```python
from build123d import *

# Parameters (mm, degrees)
SKETCH1_W           = 390
SKETCH1_H           = 756.8
BOSS_EXTRUDE1_DEPTH = 20
SKETCH2_R           = 6.05
BOSS_EXTRUDE2_DEPTH = 10
SKETCH3_R           = 6.631048811
BOSS_EXTRUDE3_DEPTH = 10
CHAMFER1_SIZE       = 10
BOSS_EXTRUDE5_DEPTH = 50
SKETCH5_W           = 30
SKETCH5_H           = 160
CUT_EXTRUDE1_DEPTH  = 50
CHAMFER2_SIZE       = 10


with BuildPart() as part:
    # Sketch1 → Boss-Extrude1 (new body)
    with BuildSketch(Plane.XY):
        with Locations((154.409313495, -346.327898551)):
            Rectangle(SKETCH1_W, SKETCH1_H)
    extrude(amount=BOSS_EXTRUDE1_DEPTH)

    # Sketch2 → Boss-Extrude2 (add)
    with BuildSketch(Plane(origin=(0, 32.072101449, 0), x_dir=(1, 0, 0), z_dir=(0, 1, 0))):
        with Locations(Location((-28.78378628, -10.435138004, 0), (0, 0, 90))):
            Circle(SKETCH2_R)
    extrude(amount=BOSS_EXTRUDE2_DEPTH)

    # Sketch3 → Boss-Extrude3 (add)
    with BuildSketch(Plane.XZ.offset(724.727898551)):
        with Locations(Location((-28.78378628, 10.435138004, 0), (0, 0, 90))):
            Circle(SKETCH3_R)
    extrude(amount=BOSS_EXTRUDE3_DEPTH)

    # Chamfer1
    # the kernel refuses this chamfer: 10 mm, written as the material it takes off along each edge
    with BuildSketch(Plane(origin=(-40.590686505, -750.44472843, 20), x_dir=(-0.027495876610586317, 0, -0.9996219169112968), z_dir=(0, 1, 0)), Plane(origin=(349.409313495, 57.788931329, 0), x_dir=(-0.9996219169112968, 0, -0.027495876610586334), z_dir=(0, -1, 0))) as chamfer1_piece_1:
        Polygon((CHAMFER1_SIZE * 0.999621916911, -CHAMFER1_SIZE * 0.0274958766106), (-CHAMFER1_SIZE * 0.0274958766106, -CHAMFER1_SIZE * 0.999621916911), (0, 0), align=None)
    extrude(amount=808.233659759, mode=Mode.SUBTRACT)
    with BuildSketch(Plane(origin=(375.126143374, -724.727898551, 20), x_dir=(0, 0.9996219169112968, 0.02749587661058643), z_dir=(-1, 0, 0))) as chamfer1_piece_2_section:
        Polygon((CHAMFER1_SIZE * 0.999621916911, CHAMFER1_SIZE * 0.0274958766106), (-CHAMFER1_SIZE * 0.0274958766106, CHAMFER1_SIZE * 0.999621916911), (0, 0), align=None)
    chamfer1_piece_2 = extrude(amount=441.433659759, mode=Mode.PRIVATE)
    chamfer1_piece_2 = chamfer1_piece_2 - Plane(origin=(-28.78378628, -721.415314621, 10.435138004), x_dir=(0, 0, 1), z_dir=(0, 1, 0)) * Cylinder(6.631048811, 923, mode=Mode.PRIVATE)
    add(chamfer1_piece_2, mode=Mode.SUBTRACT)
    with BuildSketch(Plane(origin=(349.409313495, 57.788931329, 20), x_dir=(-0.9996219169112968, 0, 0.027495876610586282), z_dir=(0, -1, 0)), Plane(origin=(-40.590686505, -750.44472843, 0), x_dir=(-0.027495876610586317, 0, 0.9996219169112968), z_dir=(0, 1, 0))) as chamfer1_piece_3:
        Polygon((CHAMFER1_SIZE * 0.999621916911, CHAMFER1_SIZE * 0.0274958766106), (-CHAMFER1_SIZE * 0.0274958766106, CHAMFER1_SIZE * 0.999621916911), (0, 0), align=None)
    extrude(amount=808.233659759, mode=Mode.SUBTRACT)
    with BuildSketch(Plane(origin=(-66.307516385, 32.072101449, 20), x_dir=(0, 0.027495876610586317, -0.9996219169112968), z_dir=(1, 0, 0))) as chamfer1_piece_4_section:
        Polygon((CHAMFER1_SIZE * 0.999621916911, -CHAMFER1_SIZE * 0.0274958766106), (-CHAMFER1_SIZE * 0.0274958766106, -CHAMFER1_SIZE * 0.999621916911), (0, 0), align=None)
    chamfer1_piece_4 = extrude(amount=441.433659759, mode=Mode.PRIVATE)
    chamfer1_piece_4 = chamfer1_piece_4 - Plane(origin=(-28.78378628, 28.76135635, 10.435138004), x_dir=(0, 0, -1), z_dir=(0, -1, 0)) * Cylinder(6.05, 923, mode=Mode.PRIVATE)
    add(chamfer1_piece_4, mode=Mode.SUBTRACT)
    with BuildSketch(Plane(origin=(375.126143374, -724.727898551, 0), x_dir=(0, 0.9996219169112968, -0.027495876610586487), z_dir=(-1, 0, 0))) as chamfer1_piece_5_section:
        Polygon((CHAMFER1_SIZE * 0.999621916911, -CHAMFER1_SIZE * 0.0274958766106), (-CHAMFER1_SIZE * 0.0274958766106, -CHAMFER1_SIZE * 0.999621916911), (0, 0), align=None)
    chamfer1_piece_5 = extrude(amount=441.433659759, mode=Mode.PRIVATE)
    chamfer1_piece_5 = chamfer1_piece_5 - Plane(origin=(-28.78378628, -721.416873801, 10.435138004), x_dir=(0, 0, 1), z_dir=(0, 1, 0)) * Cylinder(6.631048811, 923, mode=Mode.PRIVATE)
    add(chamfer1_piece_5, mode=Mode.SUBTRACT)
    with BuildSketch(Plane(origin=(-66.307516385, 32.072101449, 0), x_dir=(0, 0.027495876610586317, 0.9996219169112968), z_dir=(1, 0, 0))) as chamfer1_piece_6_section:
        Polygon((CHAMFER1_SIZE * 0.999621916911, CHAMFER1_SIZE * 0.0274958766106), (-CHAMFER1_SIZE * 0.0274958766106, CHAMFER1_SIZE * 0.999621916911), (0, 0), align=None)
    chamfer1_piece_6 = extrude(amount=441.433659759, mode=Mode.PRIVATE)
    chamfer1_piece_6 = chamfer1_piece_6 - Plane(origin=(-28.78378628, 28.763199232, 10.435138004), x_dir=(0, 0, -1), z_dir=(0, -1, 0)) * Cylinder(6.05, 923, mode=Mode.PRIVATE)
    add(chamfer1_piece_6, mode=Mode.SUBTRACT)

    # Sketch4 → Boss-Extrude5 (add)
    with BuildSketch(Plane.XY.offset(20)):
        Polygon((309.409313495, -346.327898551), (309.409313495, -246.327898551), (339.409313495, -246.327898551), (339.409313495, -446.327898551), (309.409313495, -446.327898551), align=None)
    extrude(amount=BOSS_EXTRUDE5_DEPTH)

    # Sketch5 → Cut-Extrude1 (cut)
    with BuildSketch(Plane(origin=(339.409313495, 0, 0), x_dir=(0, 0, -1), z_dir=(1, 0, 0))):
        with Locations((-35, -346.327898551)):
            Rectangle(SKETCH5_W, SKETCH5_H)
    extrude(amount=-CUT_EXTRUDE1_DEPTH, mode=Mode.SUBTRACT)

    # Chamfer2
    chamfer2_edges = [part.edges().sort_by_distance(p)[0] for p in [
        (309.409313495, -346.327898551, 70),
        (309.409313495, -246.327898551, 45),
        (324.409313495, -446.327898551, 70),
        (309.409313495, -446.327898551, 45),
        (339.409313495, -446.327898551, 45),
        (324.409313495, -246.327898551, 70),
        (339.409313495, -246.327898551, 45),
        (339.409313495, -346.327898551, 70),
    ]]
    chamfer(chamfer2_edges, length=CHAMFER2_SIZE)


solid = part.part
```
Build history of the part. All positions in model axes, mm. A direction names the side the tool comes from. Give positions to 0.01 mm unless a question says otherwise; leave off trailing zeros. Loops run counter-clockwise (first coordinate to the right, second up) from the corner with the lowest first, then second, coordinate; pieces in that order, holes last. Notation, with made-up numbers: (10.25, -36.5) -> (21.25, -36.5) arc R11 ccw to (21.25, -20.5) -> close; hole circle Ø9 at (42, 1). An arc over 180 degrees is marked (long way). One line per question, with ' | ' between items. Start each with the question number.
1) Cut at B-B (y = -305.5). Give the cut face in (x, z), plus the area to 3 significant figures.
2) 3-axis set-ups, long thin cutter, end or side, ignore diameter. For faces 5 (the flat face through (152, -341, 0)), 6 (the flat face through (325, -347, 50)), 7 (the flat face through (309.409, -339.2, 50.3)): which of +Z, -Z, +X, -X, +Y, -Y reach the whole face in a straight line?
3) Two-plate mould, pull along Y, no slides. Class faces 1 (the flat face through (325, -426.328, 35)), 2 (the flat face through (325, -266.328, 35)), 3 (the flat face through (-29, -734.728, 10)), 4 (the flat face through (339.409, -339.2, 50.3)): released by +Y, released by -Y, zero draft, split by the parting line, or undercut.
4) Pin check, flat tips, straight feed: pin 1 (5 mm diameter, centred on x = 106, y = -155, fed in from +Z); pin 2 (8 mm diameter, centred on x = 325, z = 49.5, fed in from +Y); pin 3 (2 mm diameter, centred on y = -444.5, z = 57.5, fed in from +X). Stop position of each tip, or through.
5) Cut at D-D (x = 64). Give the cut face in (y, z), plus the area to 3 significant figures.
6) Cut at A-A (z = 39). Give the cut face in (x, y), plus the area to 3 significant figures.
7) Probe L1, parallel to Y at x = 321, z = 38; L2, parallel to Z at x = 84, y = -330.5; L3, parallel to Z at x = 316.5, y = -373. List the from-to ranges inside material, lowest first.
8) Cut at C-C (y = -648.5). Give the cut face in (x, z), plus the area to 3 significant figures.
Return value:
1) outline: (-40.59, 10) -> (-30.59, 0) -> (339.41, 0) -> (349.41, 10) -> (339.41, 20) -> (-30.59, 20) -> close; (309.41, 50) -> (339.41, 50) -> (339.41, 60) -> (329.41, 70) -> (319.41, 70) -> (309.41, 60) -> close | area: 8,100 mm^2
2) face 5: -Z, +X, -X, +Y, -Y | face 6: +X, -X | face 7: +Z, -X, +Y, -Y
3) face 1: undercut | face 2: undercut | face 3: released by -Y | face 4: zero draft
4) pin 1: z = 20 | pin 2: y = -246.33 | pin 3: x = 332.24
5) outline: (-724.73, 10) -> (-714.73, 0) -> (22.07, 0) -> (32.07, 10) -> (22.07, 20) -> (-714.73, 20) -> close | area: 14,900 mm^2
6) outline: (309.41, -436.33) -> (319.41, -446.33) -> (329.41, -446.33) -> (339.41, -436.33) -> (339.41, -426.33) -> (309.41, -426.33) -> close; (309.41, -266.33) -> (339.41, -266.33) -> (339.41, -256.33) -> (329.41, -246.33) -> (319.41, -246.33) -> (309.41, -256.33) -> close | area: 1,000 mm^2
7) L1: -446.33 to -426.33, -266.33 to -246.33 | L2: 0 to 20 | L3: 0 to 20, 50 to 67.09
8) outline: (-40.59, 10) -> (-30.59, 0) -> (339.41, 0) -> (349.41, 10) -> (339.41, 20) -> (-30.59, 20) -> close | area: 7,600 mm^2
